The model under review builds one solid part; all positions refer to its coordinate system, in mm. A direction names the side the tool comes from. Round coordinates to 2 decimals unless told otherwise and drop trailing zeros. Write each loop counter-clockwise with the first axis right and the second up, starting at its lowest first coordinate (ties: lowest second). Pieces come first, ordered by that corner, then holes. Notation, with made-up numbers: (49, 62.5) - (69, 62.5) arc R18 cw to (69, 94.5) - close; hole circle Ø7 at (-15.5, -3). An arc over 180 degrees is marked (long way). Return JSON: item names as keys, results as strings.
from build123d import *

# Parameters (mm, degrees)
BOSS_EXTRUDE1_DEPTH            = 44
CBORE_FOR_M3_SHCS1_D           = 3.4
CBORE_FOR_M3_SHCS1_CBORE_D     = 6.5
CBORE_FOR_M3_SHCS1_CBORE_DEPTH = 3
CIRPATTERN1_COUNT              = 4
SKETCH4_R                      = 16.2
CUT_EXTRUDE1_DEPTH             = 35
SKETCH5_R                      = 8
CUT_EXTRUDE2_DEPTH             = 67.748127315
BOSS_EXTRUDE2_DEPTH            = 44
CBORE_FOR_M4_SHCS1_D           = 4.3
CBORE_FOR_M4_SHCS1_DEPTH       = 100.101198794
CBORE_FOR_M4_SHCS1_CBORE_D     = 8
CBORE_FOR_M4_SHCS1_CBORE_DEPTH = 4
CBORE_FOR_M4_SHCS1_TIP         = 1.291850331


with BuildPart() as part:
    # Sketch1 → Boss-Extrude1 (new body)
    with BuildSketch(Plane(origin=(0, 0, 0), x_dir=(1, 0, 0), z_dir=(0, 1, 0))):
        with BuildLine():
            Line((-32.5, 20.169593452), (-32.5, -20.169593452))
            ThreePointArc((-32.5, -20.169593452), (0, -38.25), (32.5, -20.169593452))
            Line((32.5, -20.169593452), (32.5, 20.169593452))
            ThreePointArc((32.5, 20.169593452), (0, 38.25), (-32.5, 20.169593452))
        make_face()
    extrude(amount=BOSS_EXTRUDE1_DEPTH)

    # CBORE for M3 SHCS1 (through all)
    with Locations(Plane(origin=(0, 44, 0), x_dir=(1, 0, 0), z_dir=(0, 1, 0))):
        with Locations((-4.446261863, 12.21600407)):
            cbore_for_m3_shcs1 = CounterBoreHole(CBORE_FOR_M3_SHCS1_D / 2, CBORE_FOR_M3_SHCS1_CBORE_D / 2, CBORE_FOR_M3_SHCS1_CBORE_DEPTH)

    # CirPattern1: CBORE for M3 SHCS1 ×4 about axis
    cirpattern1_axis = Axis((0, 0, 0), (0, 1, 0))
    for i in range(1, CIRPATTERN1_COUNT):
        add(cbore_for_m3_shcs1.rotate(cirpattern1_axis, i * 360 / CIRPATTERN1_COUNT), mode=Mode.SUBTRACT)

    # Sketch4 → Cut-Extrude1 (cut)
    with BuildSketch(Plane.XZ):
        with Locations(Location((0, 0, 0), (0, 0, 270))):
            Circle(SKETCH4_R)
    extrude(amount=-CUT_EXTRUDE1_DEPTH, mode=Mode.SUBTRACT)

    # Sketch5 → Cut-Extrude2 (cut, through all)
    with BuildSketch(Plane(origin=(0, 44, 0), x_dir=(1, 0, 0), z_dir=(0, 1, 0))):
        with Locations(Location((0, 0, 0), (0, 0, 270))):
            Circle(SKETCH5_R)
    extrude(amount=-CUT_EXTRUDE2_DEPTH, mode=Mode.SUBTRACT)

    # Sketch7 → Boss-Extrude2 (add)
    with BuildSketch(Plane.XZ):
        with BuildLine():
            Line((-32.5, 20.169593452), (-32.5, 22.007101127))
            ThreePointArc((-32.5, 22.007101127), (0, 39.25), (32.5, 22.007101127))
            Line((32.5, 22.007101127), (32.5, 20.169593452))
            ThreePointArc((32.5, 20.169593452), (0, 38.25), (-32.5, 20.169593452))
        make_face()
        with BuildLine():
            Line((32.5, -20.169593452), (32.5, -22.007101127))
            ThreePointArc((32.5, -22.007101127), (0, -39.25), (-32.5, -22.007101127))
            Line((-32.5, -22.007101127), (-32.5, -20.169593452))
            ThreePointArc((-32.5, -20.169593452), (0, -38.25), (32.5, -20.169593452))
        make_face()
    extrude(amount=-BOSS_EXTRUDE2_DEPTH)

    # CBORE for M4 SHCS1
    with Locations(Plane(origin=(-50.050599397, 499.724238547, -401.677021233), x_dir=(0, -0.9858598075393219, -0.16757219303491563), z_dir=(-1, 0, 0))):
        with Locations((405.876811742, 451.068889591), (423.622288278, 454.085189065)):
            CounterBoreHole(CBORE_FOR_M4_SHCS1_D / 2, CBORE_FOR_M4_SHCS1_CBORE_D / 2, CBORE_FOR_M4_SHCS1_CBORE_DEPTH, depth=CBORE_FOR_M4_SHCS1_DEPTH)
            with Locations((0, 0, -(CBORE_FOR_M4_SHCS1_DEPTH + CBORE_FOR_M4_SHCS1_TIP / 2))):  # 118° drill point
                Cone(0, CBORE_FOR_M4_SHCS1_D / 2, CBORE_FOR_M4_SHCS1_TIP, mode=Mode.SUBTRACT)


solid = part.part
(1) Wall thickness on line 1 (X direction, y = 19.5, z = 0); line 2 (Y direction, x = -6, z = 13); line 3 (X direction, y = 41, z = 0): over which ranges is each line inside the solid? List them lowest first.
Filled in:
{"line 1": "x = -32.5 to -16.2, 16.2 to 32.5", "line 2": "y = 35 to 44", "line 3": "x = -32.5 to -8, 8 to 32.5"}
(2) Mouldability with a two-part tool opening along X and no side actions: class faces 4 (the cylindrical face through (-0.536, 21.692, 39.246)), 5 (the cylindrical face through (2.748, 37.958, 12.291)), 6 (the cylindrical face through (13.36, 37.96, -3.19)), 7 (the flat face through (0.5, 44, -8.2)) as released by +X, released by -X, zero draft, split by the parting line, or undercut.
Filled in:
{"face 4": "split by the parting line", "face 5": "undercut", "face 6": "undercut", "face 7": "zero draft"}
(3) Add section C-C (x = 0). Write out the cut boundary in (y, z), plus the area to 3 significant figures.
Filled in:
{"outline": "(0, -39.25) - (44, -39.25) - (44, -8) - (35, -8) - (35, -16.2) - (0, -16.2) - close; (0, 16.2) - (35, 16.2) - (35, 8) - (44, 8) - (44, 39.25) - (0, 39.25) - close; hole circle Ø4.3 at (6, -25); hole circle Ø4.3 at (24, -25)", "area": "2,150 mm2"}
(4) Add section B-B (z = 0). Write out the cut boundary in (x, y).
Filled in:
{"outline": "(-32.5, 0) - (-16.2, 0) - (-16.2, 35) - (-8, 35) - (-8, 44) - (-32.5, 44) - close; (8, 35) - (16.2, 35) - (16.2, 0) - (32.5, 0) - (32.5, 44) - (8, 44) - close"}
(5) Add section A-A (y = 7). Write out the cut boundary in (x, z), plus the area to 3 significant figures.
Filled in:
{"outline": "(-32.5, -22.01) arc R39.25 ccw to (-31.73, -23.1) - (31.73, -23.1) arc R39.25 ccw to (32.5, -22.01) - (32.5, 22.01) arc R39.25 ccw to (-32.5, 22.01) - close; (-28.58, -26.9) arc R39.25 ccw to (28.58, -26.9) - close; hole circle Ø32.4 at (0, 0)", "area": "3,380 mm2"}
(6) Add section D-D (y = 14.5). Write out the cut boundary in (x, z).
Filled in:
{"outline": "(-32.5, -22.01) arc R39.25 ccw to (32.5, -22.01) - (32.5, 22.01) arc R39.25 ccw to (-32.5, 22.01) - close; hole circle Ø32.4 at (0, 0)"}
(7) Clearance check with flat-ended pins moving along their axes: pin 1 Ø12 at (y, z) = (14, 31) entering from -X; pin 2 Ø1 at (x, z) = (-3, 9) entering from -Y; pin 3 Ø4 at (x, z) = (-4.45, -12.22) entering from +Y; pin 4 Ø3 at (x, z) = (4.45, 12.22) entering from +Y. State where each tip first meets the part, or that it passes through.
Filled in:
{"pin 1": "stops at x = -30.26", "pin 2": "stops at y = 35", "pin 3": "stops at y = 41", "pin 4": "passes through"}
(8) For faces 1 (the flat face through (11, 41, -3)), 2 (the cylindrical face through (-2.748, 37.958, -12.291)), 3 (the cylindrical face through (-14.37, 17.26, -7.48)), list the 3-axis set-ups (+Z, -Z, +X, -X, +Y, -Y) from which the entire face can be reached by the end or side of a thin tool; tool diameter is ignored.
Filled in:
{"face 1": "+Y", "face 2": "+Y, -Y", "face 3": "-Y"}
